Can you work these out from the drawing? Everything is in mm from the part's minimum corner. Coordinates: 2 decimals unless noted, no trailing zeros. Write each loop counter-clockwise with the first axis right and the second up, starting at its lowest first coordinate (ties: lowest second). Pieces come first, ordered by that corner, then holes. Notation, with made-up numbers: M 15,52.5 L 64,52.5 A23 cw 64,91.5 Z; hole C 38,71 d9. An arc over 180 degrees is marked long. Write item = value, one per line.
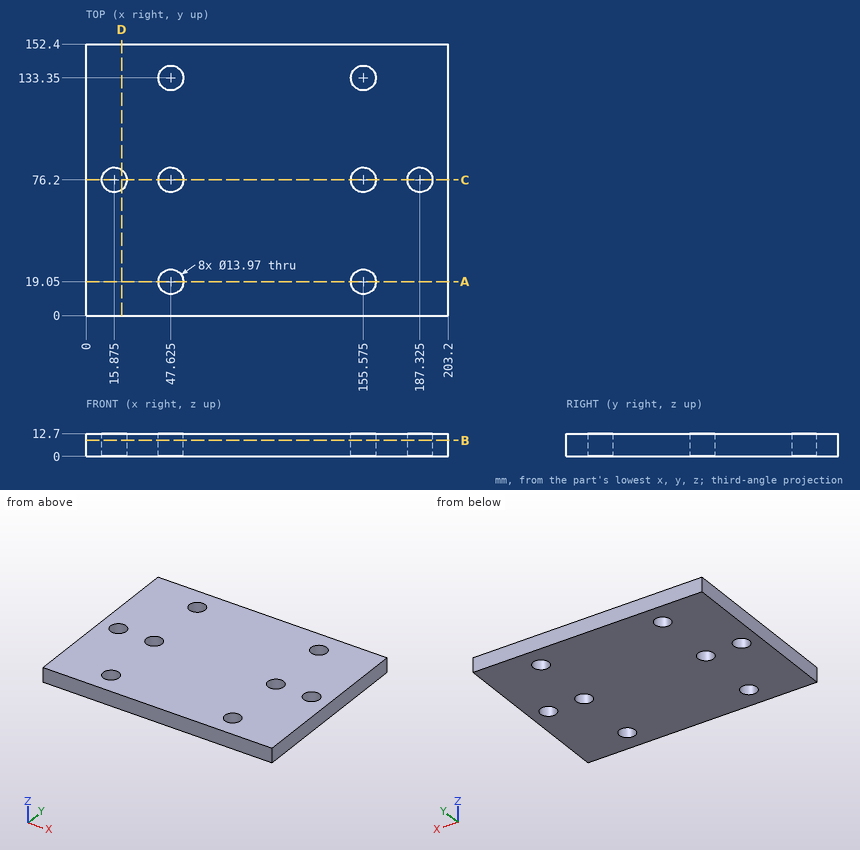
Item 1: Imagine slicing it at A-A (y = 19.05). Write out the boundary of the cut face in (x, z).
Numbers:
outline = M 0,0 L 40.64,0 L 40.64,12.7 L 0,12.7 Z; M 54.61,0 L 148.59,0 L 148.59,12.7 L 54.61,12.7 Z; M 162.56,0 L 203.2,0 L 203.2,12.7 L 162.56,12.7 Z
Item 2: If I drill on line 1 along Y through (x, z) = (157, 9.5); line 2 along Y through (x, z) = (10.5, 2.75); line 3 along X through (y, z) = (78.5, 4.5), over which ranges is the centre line in solid material (lowest first)?
Numbers:
line_1 = 0 to 12.21, 25.89 to 69.36, 83.04 to 126.51, 140.19 to 152.4
line_2 = 0 to 71.74, 80.66 to 152.4
line_3 = 0 to 9.28, 22.47 to 41.03, 54.22 to 148.98, 162.17 to 180.73, 193.92 to 203.2
Item 3: Imagine slicing it at D-D (x = 20). Write out the boundary of the cut face in (y, z), and give its area (3 significant figures).
Numbers:
outline = M 0,0 L 70.56,0 L 70.56,12.7 L 0,12.7 Z; M 81.84,0 L 152.4,0 L 152.4,12.7 L 81.84,12.7 Z
area = 1,790 mm²
Item 4: Imagine slicing it at C-C (y = 76.2). Write out the boundary of the cut face in (x, z), and give its area (3 significant figures).
Numbers:
outline = M 0,0 L 8.89,0 L 8.89,12.7 L 0,12.7 Z; M 22.86,0 L 40.64,0 L 40.64,12.7 L 22.86,12.7 Z; M 54.61,0 L 148.59,0 L 148.59,12.7 L 54.61,12.7 Z; M 162.56,0 L 180.34,0 L 180.34,12.7 L 162.56,12.7 Z; M 194.31,0 L 203.2,0 L 203.2,12.7 L 194.31,12.7 Z
area = 1,870 mm²
Item 5: Imagine slicing it at B-B (z = 9). State how many separate pieces and enclosed holes the cut face has, and give its area (3 significant figures).
Numbers:
separate_pieces = 1
enclosed_holes = 8
area = 29,700 mm²
